Read the model definition and answer for the solid it produces. Units are mm, in the model's axes. Face numbers are marked on the shaded views. A direction names the side the tool comes from. Coordinates: 2 decimals unless noted, no trailing zeros. Order: outer loops, then holes, each group sorted by start corner. A loop starts at its lowest first (then second) coordinate and runs counter-clockwise, first axis right, second up. Notation, with made-up numbers: (-31.75, 76) -> (9.25, 76) arc R32 cw to (9.25, 106) -> close; hole circle Ø6 at (60, 15). An arc over 180 degrees is marked (long way). Return JSON: item names as keys, results as strings. Group by question number.
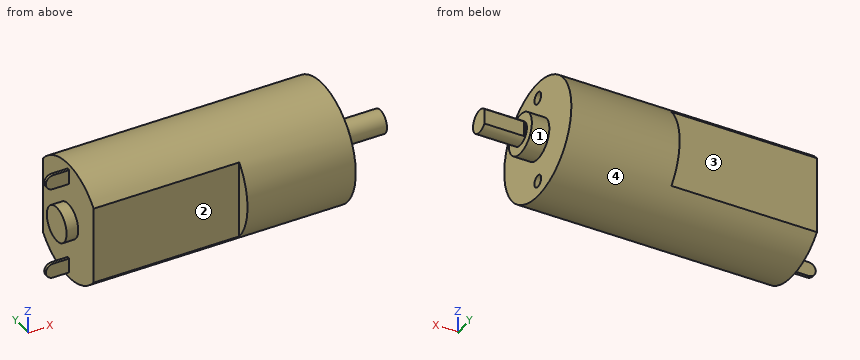
```python
from build123d import *

# Parameters (mm, degrees)
CUT_EXTRUDE1_START           = -6.8
CUT_EXTRUDE1_DEPTH           = 6.8
CUT_EXTRUDE2_DEPTH           = 25
M2_5X0_45_TAPPED_HOLE1_D     = 2.05
M2_5X0_45_TAPPED_HOLE1_DEPTH = 6.35
M2_5X0_45_TAPPED_HOLE1_TIP   = 0.615882135
BOSS_EXTRUDE1_DEPTH          = 0.25
SKETCH8_R                    = 3
BOSS_EXTRUDE2_DEPTH          = 2


with BuildPart() as part:
    # Sketch1 → Revolve1 (revolve)
    with BuildSketch(Plane.XY, mode=Mode.PRIVATE) as revolve1_sk:
        Polygon((-26.8, 0), (26.8, 0), (26.8, 2), (19.8, 2), (19.8, 3.5), (16.8, 3.5), (16.8, 10.2), (-26.8, 10.2), align=None)
    revolve(revolve1_sk.sketch.rotate(Axis((-26.8, 0, 0), (1, 0, 0)), 90), axis=Axis((-26.8, 0, 0), (1, 0, 0)))

    # Sketch3 → Cut-Extrude1 (cut)
    with BuildSketch(Plane(origin=(26.8, 0, 0), x_dir=(0, 0, -1), z_dir=(1, 0, 0)).offset(CUT_EXTRUDE1_START)):
        with BuildLine():
            Line((-1.322875656, 1.5), (1.322875656, 1.5))
            ThreePointArc((1.322875656, 1.5), (0, 2), (-1.322875656, 1.5))
        make_face()
    extrude(amount=CUT_EXTRUDE1_DEPTH, mode=Mode.SUBTRACT)

    # Sketch4 → Cut-Extrude2 (cut)
    with BuildSketch(Plane.ZY.offset(26.8)):
        with BuildLine():
            Line((-6.68954408, 7.7), (6.68954408, 7.7))
            ThreePointArc((6.68954408, 7.7), (0, 10.2), (-6.68954408, 7.7))
        make_face()
        with BuildLine():
            Line((-6.68954408, -7.7), (6.68954408, -7.7))
            ThreePointArc((6.68954408, -7.7), (0, -10.2), (-6.68954408, -7.7))
        make_face()
    extrude(amount=-CUT_EXTRUDE2_DEPTH, mode=Mode.SUBTRACT)

    # M2.5x0.45 Tapped Hole1
    with Locations(Plane(origin=(16.8, 0, 0), x_dir=(0, 0, -1), z_dir=(1, 0, 0))):
        with Locations((-7.5, 0), (7.5, 0)):
            Hole(M2_5X0_45_TAPPED_HOLE1_D / 2, depth=M2_5X0_45_TAPPED_HOLE1_DEPTH)
            with Locations((0, 0, -(M2_5X0_45_TAPPED_HOLE1_DEPTH + M2_5X0_45_TAPPED_HOLE1_TIP / 2))):  # 118° drill point
                Cone(0, M2_5X0_45_TAPPED_HOLE1_D / 2, M2_5X0_45_TAPPED_HOLE1_TIP, mode=Mode.SUBTRACT)

    # Sketch7 → Boss-Extrude1 (add, symmetric)
    with BuildSketch(Plane(origin=(0, 0, 0), x_dir=(1, 0, 0), z_dir=(0, 1, 0))):
        with BuildLine():
            Line((-26.8, 9.25), (-29.55, 9.25))
            ThreePointArc((-29.55, 9.25), (-30.8, 8), (-29.55, 6.75))
            Line((-29.55, 6.75), (-26.8, 6.75))
            Line((-26.8, 6.75), (-26.8, 9.25))
        make_face()
        with BuildLine():
            Line((-26.8, -6.75), (-26.8, -9.25))
            Line((-26.8, -9.25), (-29.55, -9.25))
            ThreePointArc((-29.55, -9.25), (-30.8, -8), (-29.55, -6.75))
            Line((-29.55, -6.75), (-26.8, -6.75))
        make_face()
    extrude(amount=BOSS_EXTRUDE1_DEPTH, both=True)

    # Sketch8 → Boss-Extrude2 (add)
    with BuildSketch(Plane.ZY.offset(26.8)):
        with Locations(Location((0, 0, 0), (0, 0, 180))):
            Circle(SKETCH8_R)
    extrude(amount=BOSS_EXTRUDE2_DEPTH)


solid = part.part
```
1. Find section D-D on y = -5. Determine the outline of the cut face in (x, z).
2. Find section B-B on x = -1. Determine the outline of the cut face in (y, z).
3. Find section C-C on x = 15.5. Determine the outline of the cut face in (y, z) (3 decimals), and give its area (3 significant figures).
4. Given pin 1 (4 mm diameter, centred on y = -6.5, z = -6, fed in from -X); pin 2 (5 mm diameter, centred on x = -5.5, z = -0.5, fed in from +Y); pin 3 (1.3 mm diameter, centred on x = 22, z = -0.5, fed in from +Y), each flat-ended and moving along its own axis, determine where each tip first touches the part or whether it passes through.
5. Find section A-A on z = 0. Determine the outline of the cut face in (x, y).
6. Straight lines are drawn through the part: L1, parallel to Y at x = -13.5, z = -5; L2, parallel to X at y = 0.5, z = 0.5; L3, parallel to X at y = 1.5, z = 8. For each, find the intervals that lie inside material, in ascending order.
7. Which of the six approach directions +Z, -Z, +X, -X, +Y, -Y give full straight-line access (tool end or side, diameter ignored) to the marked faces 1, 2, 3 and 4?
Result:
{
 "1": {"outline": "(-26.8, -8.89) -> (16.8, -8.89) -> (16.8, 8.89) -> (-26.8, 8.89) -> close"},
 "2": {"outline": "circle Ø20.4 at (0, 0)"},
 "3": {"outline": "circle Ø20.4 at (0, 0); hole circle Ø2.05 at (0, -7.5); hole circle Ø2.05 at (0, 7.5)", "area": "320 mm^2"},
 "4": {"pin 1": "x = -26.8", "pin 2": "y = 7.7", "pin 3": "y = 1.5"},
 "5": {"outline": "(-28.8, -3) -> (-26.8, -3) -> (-26.8, -7.7) -> (-1.8, -7.7) -> (-1.8, -10.2) -> (16.8, -10.2) -> (16.8, -3.5) -> (19.8, -3.5) -> (19.8, -2) -> (26.8, -2) -> (26.8, 1.5) -> (20, 1.5) -> (20, 2) -> (19.8, 2) -> (19.8, 3.5) -> (16.8, 3.5) -> (16.8, 10.2) -> (-1.8, 10.2) -> (-1.8, 7.7) -> (-26.8, 7.7) -> (-26.8, 3) -> (-28.8, 3) -> close"},
 "6": {"L1": "-7.7 to 7.7", "L2": "-28.8 to 26.8", "L3": "-26.8 to 16.8"},
 "7": {"face 1": "+X", "face 2": "+Z, -Z, -X, -Y", "face 3": "+Z, -Z, -X, +Y", "face 4": "+X, -X"}
}
